Autodesk Inventor part; units mm, degrees
ref_plane "XZ Plane" through (0, 0, 0) normal (0, 1, 0) x (-1, 0, 0)
ref_plane "XY Plane" through (0, 0, 0) normal (0, 0, 1) x (1, 0, 0)
sketch "Sketch1" plane through (0, 0, 0) normal (0, 1, 0) x (-1, 0, 0)
  line L0 (-12.7, 12.7) -> (-12.7, -12.7)
  line L1 (-12.7, -12.7) -> (12.7, -12.7)
  line L2 (12.7, -12.7) -> (12.7, 12.7)
  line L3 (12.7, 12.7) -> (-12.7, 12.7)
  line L4 (-12.7, 12.7) -> (12.7, -12.7) construction
  line L5 (-12.7, -12.7) -> (12.7, 12.7) construction
  point P0 (0, 0)
  dimension "d0" = 25.4
extrude "Extrusion1" add sketch "Sketch1" along normal blind 101.6
sketch "Sketch3" plane through (-12.7, 0, -12.7) normal (-1, 0, 0) x (0, 0, 1)
  line L0 (25.4, 101.6) -> (0, 101.6)
  line L1 (0, 101.6) -> (25.4, 101.6)
  line L2 (25.4, 101.6) -> (25.4, 77.8642)
  line L3 (25.4, 77.8642) -> (0, 77.8642)
  line L4 (0, 77.8642) -> (0, 101.6)
  point P0 (12.7, 0)
extrude "Extrusion3" add sketch "Sketch3" along normal blind 50.8
sketch "Sketch4" plane through (-12.7, 0, 12.7) normal (0, 0, 1) x (1, 0, 0)
  line L0 (25.4, 0) -> (25.4, 101.6)
  line L1 (25.4, 101.6) -> (61.321, 137.521)
  line L2 (25.4, 101.6) -> (76.2, 101.6) construction
  line L3 (61.321, 137.521) -> (76.8907, 121.9514)
  line L4 (76.8907, 121.9514) -> (25.4, 70.4607)
  point P0 (12.7, 0)
  dimension "d7" = 50.8
  dimension "d8" = 45
extrude "Extrusion4" add sketch "Sketch4" against normal blind 25.4
ref_plane "Work Plane2" through (-12.7, 77.8642, -12.7) normal (0.766, -0.6428, 0) x (0, 0, -1)
sketch "Sketch6" plane through (-12.7, 77.8642, -12.7) normal (0.766, -0.6428, 0) x (0, 0, -1)
  line L0 (0, 83.1971) -> (0, 10.6554)
  line L1 (-25.4, 10.6554) -> (-25.4, 83.1971)
  line L2 (0, 30.9038) -> (-25.4, 30.9038)
  line L3 (-25.4, 30.9038) -> (-25.4, 13.0904)
  line L4 (-25.4, 13.0904) -> (0, 13.0904)
  line L5 (0, 13.0904) -> (0, 30.9038)
  point P0 (-12.7, -51.4841)
  point P1 (0, 13.0904)
  point P2 (-25.4, 30.9038)
extrude "Extrusion6" add sketch "Sketch6" against normal blind 101.6
sketch "Sketch7" plane through (-12.7, 77.8642, -12.7) normal (0.766, -0.6428, 0) x (0, 0, -1)
  point P0 (-12.7, -51.4841)
properties part number "example01"
Here's how the part is built. I have some questions about the finished solid (model axes, mm). A direction names the side the tool comes from. Round coordinates to 2 decimals unless told otherwise and drop trailing zeros. Order: outer loops, then holes, each group sorted by start corner. A loop starts at its lowest first (then second) coordinate and runs counter-clockwise, first axis right, second up. Notation, with made-up numbers: M 21,37 L 32,37 A4 cw 32,43 Z; hole C -35,-4.75 d8. An arc over 180 degrees is marked long. Return JSON: item names as keys, results as strings. Group by question number.
1. I'm going to push flat-ended pins straight in: pin 1 Ø6 at (x, z) = (19.5, -1) entering from -Y; pin 2 Ø12.5 at (x, z) = (-33.5, 5) entering from -Y; pin 3 Ø10 at (y, z) = (29.5, 7) entering from -X. Where does each tip first touch, or does it pass through?
2. On a 3-axis mill with a long thin cutter (end or side, diameter ignored), from which of +Z, -Z, +X, -X, +Y, -Y can I reach the whole of each face in a straight line? I mean faces 1 (the face through (-31.243, 133.766, -0.178)), 2 (the face through (12.7, 35, 0)), 3 (the face through (-38, 77.864, 0)). Say none if no direction works.
3. Please list where these lines run through material, in increasing order: probe 1 along X at (y, z) = (48.5, 6); probe 2 along Y at (x, z) = (-38.5, -1.25); probe 3 along Y at (x, z) = (-46.5, -2).
4. If we section it at B-B on y = 134.5: List the corners of the cut face in (x, z) for me, then the cut area to 3 significant figures.
5. If we mould it in two halves opening along X, with no side actions, what happens to faces 4 (the face through (30.4, 119.3, 0.2)), 5 (the face through (-9, 90, 12.7)), 6 (the face through (-50.94, 127.04, 0.18))? For each: pulls with the +X half, pulls with the -X half, needs draft (parallel to the pull), parting line crosses it, or undercut.
6. If we section it at D-D on y = 38: List the corners of the cut face in (x, z) for me, then the cut area to 3 significant figures.
7. If we section it at C-C on z = 5: List the corners of the cut face in (x, y) for me, then the cut area to 3 significant figures.
8. If we section it at A-A on x = -60.5: List the corners of the cut face in (y, z) for me.
Reply:
{
 "1": {"pin 1": "y = 74.26", "pin 2": "y = 77.86", "pin 3": "x = -12.7"},
 "2": {"face 1": "+Z, -Z, +Y", "face 2": "+Z, -Z, +X, -Y", "face 3": "+Z, -Z, -X, -Y"},
 "3": {"probe 1": "-12.7 to 12.7", "probe 2": "77.86 to 101.6, 116.6 to 139.86", "probe 3": "77.86 to 101.6, 123.31 to 146.57"},
 "4": {"outline": "M -59.83,-12.7 L -32.12,-12.7 L -32.12,12.7 L -59.83,12.7 Z; M 45.6,-12.7 L 51.64,-12.7 L 51.64,12.7 L 45.6,12.7 Z", "area": "857 mm^2"},
 "5": {"face 4": "undercut", "face 5": "needs draft", "face 6": "pulls with the -X half"},
 "6": {"outline": "M -12.7,-12.7 L 12.7,-12.7 L 12.7,12.7 L -12.7,12.7 Z", "area": "645 mm^2"},
 "7": {"outline": "M -82.12,153.2 L -20.62,101.6 L -63.5,101.6 L -63.5,77.86 L -12.7,77.86 L -12.7,0 L 12.7,0 L 12.7,70.46 L 64.19,121.95 L 48.62,137.52 L 12.7,101.6 L 7.09,101.6 L -70.67,166.85 Z", "area": "6,770 mm^2"},
 "8": {"outline": "M 77.86,-12.7 L 101.6,-12.7 L 101.6,12.7 L 77.86,12.7 Z; M 135.06,-12.7 L 158.32,-12.7 L 158.32,12.7 L 135.06,12.7 Z"}
}
